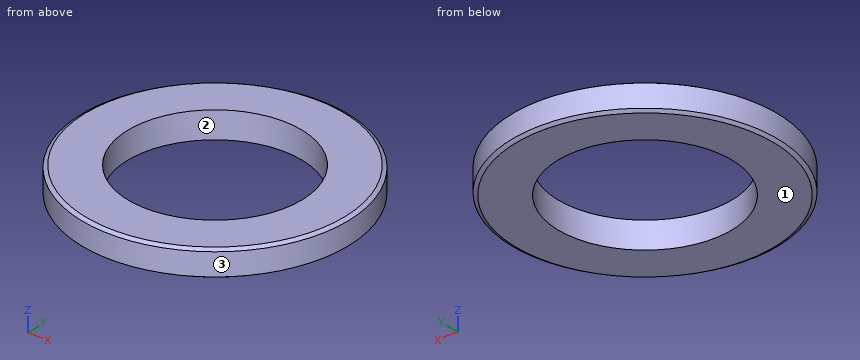
from build123d import *

# Parameters (mm, degrees)
SKETCH3_R                = 15.875
SKETCH3_R_2              = 9.5504
BOSS_EXTRUDE1_DEPTH      = 1.5875
BOSS_EXTRUDE1_DEPTH_BACK = 1.5875
CHAMFER1_SIZE            = 0.254
CHAMFER1_SIZE2           = 0.439940905
CHAMFER1_PART_2_SIZE     = 0.254
CHAMFER1_PART_2_SIZE2    = 0.439940905
CHAMFER2_SIZE            = 0.254
CHAMFER2_SIZE2           = 0.495866606
SKETCH5_R                = 10.380999939
CUT_EXTRUDE1_DEPTH       = 4.1750001


with BuildPart() as part:
    # Sketch3 → Boss-Extrude1 (new body, two sides)
    with BuildSketch(Plane.XY) as boss_extrude1_sk:
        Circle(SKETCH3_R)
        Circle(SKETCH3_R_2, mode=Mode.SUBTRACT)
    extrude(amount=BOSS_EXTRUDE1_DEPTH)
    extrude(boss_extrude1_sk.sketch, amount=-BOSS_EXTRUDE1_DEPTH_BACK)

    # Chamfer1
    chamfer1_edges = [part.edges().sort_by_distance(p)[0] for p in [
        (-15.875, 0, 1.5875),
    ]]
    chamfer1_side = [part.faces().sort_by_distance(p)[0] for p in [
        (-15.875, 0, 0.79375),
    ]]
    chamfer(chamfer1_edges, length=CHAMFER1_SIZE, length2=CHAMFER1_SIZE2, reference=chamfer1_side[0])

    # Chamfer1 part 2
    chamfer1_part_2_edges = [part.edges().sort_by_distance(p)[0] for p in [
        (-15.875, 0, -1.5875),
    ]]
    chamfer1_part_2_side = [part.faces().sort_by_distance(p)[0] for p in [
        (-15.875, 0, -0.79375),
    ]]
    chamfer(chamfer1_part_2_edges, length=CHAMFER1_PART_2_SIZE, length2=CHAMFER1_PART_2_SIZE2, reference=chamfer1_part_2_side[0])

    # Sketch4 → Cut-Revolve1 (revolve, cut)
    with BuildSketch(Plane(origin=(0, 0, 0), x_dir=(0, 0, -1), z_dir=(1, 0, 0))):
        with BuildLine():
            Line((-1.5875, 9.4996), (-1.5875, 9.6012))
            ThreePointArc((-1.5875, 9.6012), (0, 9.5504), (1.5875, 9.6012))
            Line((1.5875, 9.6012), (1.5875, 9.4996))
            Line((1.5875, 9.4996), (-1.5875, 9.4996))
        make_face()
    revolve(axis=Axis((0, 0, 1.5875), (0, 0, -1)), mode=Mode.SUBTRACT)

    # Chamfer2
    chamfer2_edges = [part.edges().sort_by_distance(p)[0] for p in [
        (0, -9.6012, -1.5875),
        (0, -9.6012, 1.5875),
    ]]
    chamfer2_side = [part.faces().sort_by_distance(p)[0] for p in [
        (0, -9.5504, 0),
    ]]
    chamfer(chamfer2_edges, length=CHAMFER2_SIZE, length2=CHAMFER2_SIZE2, reference=chamfer2_side[0])

    # Sketch5 → Cut-Extrude1 (cut, through all)
    with BuildSketch(Plane.XY.offset(1.5875)):
        Circle(SKETCH5_R)
    extrude(amount=-CUT_EXTRUDE1_DEPTH, mode=Mode.SUBTRACT)


solid = part.part
Part model, mm, in its own coordinate system. Face numbers are marked on the shaded views. Round coordinates to 2 decimals unless told otherwise and drop trailing zeros. Order: outer loops, then holes, each group sorted by start corner. A loop starts at its lowest first (then second) coordinate and runs counter-clockwise, first axis right, second up. Notation, with made-up numbers: (-24, 68.25) -> (20, 68.25) arc R13 ccw to (20, 83.25) -> close; hole circle Ø1 at (34, -20). An arc over 180 degrees is marked (long way). Put each result on its own line as item: value.
Q1. Band-saw the part on A-A (x = 0). Give the cut face in (y, z) (1 decimal).
From the geometry:
outline: (-15.9, -1.3) -> (-15.4, -1.6) -> (-10.4, -1.6) -> (-10.4, 1.6) -> (-15.4, 1.6) -> (-15.9, 1.3) -> close; (10.4, -1.6) -> (15.4, -1.6) -> (15.9, -1.3) -> (15.9, 1.3) -> (15.4, 1.6) -> (10.4, 1.6) -> close
Q2. Band-saw the part on C-C (z = -0.1). Give the cut face in (x, y) (3 decimals), and give its area (3 significant figures).
From the geometry:
outline: circle Ø31.75 at (0, 0); hole circle Ø20.762 at (0, 0)
area: 453 mm2
Q3. Wall check: line 1 (Y direction, x = 0, z = -0.15) (3 decimals); line 2 (X direction, y = -5, z = -0.3); line 3 (X direction, y = 7, z = -0.45). Give the ranges that are in metal, low to high. Write a range as [from, to].
From the geometry:
line 1: y = [-15.875, -10.381], [10.381, 15.875]
line 2: x = [-15.07, -9.1], [9.1, 15.07]
line 3: x = [-14.25, -7.67], [7.67, 14.25]
Q4. Pull direction X, two halves, no side cores. Call the marked faces 1, 2 and 3: pulls with the +X half, pulls with the -X half, needs draft (parallel to the pull), parting line crosses it, or undercut.
From the geometry:
face 1: needs draft
face 2: undercut
face 3: parting line crosses it
